Autodesk Inventor part; units mm, degrees
ref_plane "BODY_N_XY" through (79, 0, 0) normal (0, 0, -1) x (1, 0, 0)
ref_plane "BODY_N_YZ" through (79, 0, 0) normal (1, 0, 0) x (0, -1, 0)
ref_plane "BODY_N_ZX" through (79, 0, 0) normal (0, -1, 0) x (0, 0, -1)
sketch "Sketch_8" plane through (0, 0, 0) normal (0, 0, 1) x (1, 0, 0)
  line L0 (0, 0) -> (-8, 0)
  line L1 (-8, 0) -> (-8, 3.3865)
  line L2 (-8, 3.3865) -> (-7.3865, 4)
  line L3 (-7.3865, 4) -> (0, 4)
  line L4 (0, 4) -> (0, 0)
  line L5 (0, 0) -> (-8, 0)
revolve "Revolution1" add sketch "Sketch_8" angle 360 about axis through (0, 0, 0) along (1, 0, 0)
thread "Thread1"
sketch "Sketch_9" plane through (0, 0, 0) normal (1, 0, 0) x (0, 0, -1)
  line L0 (-6, 3.6056) -> (-6, -3.6056)
  arc A0 (-6, -3.6056) -> (-3.6056, -6) centre (0, 0) ccw
  line L1 (-3.6056, -6) -> (3.6056, -6)
  arc A1 (3.6056, -6) -> (6, -3.6056) centre (0, 0) ccw
  line L2 (6, -3.6056) -> (6, 3.6056)
  arc A2 (6, 3.6056) -> (3.6056, 6) centre (0, 0) ccw
  line L3 (3.6056, 6) -> (-3.6056, 6)
  arc A3 (-3.6056, 6) -> (-6, 3.6056) centre (0, 0) ccw
extrude "Extrusion1" add sketch "Sketch_9" along normal blind 12.5
sketch "Sketch_6" plane through (12.5, 0, 0) normal (1, 0, 0) x (0, 0, -1)
  circle A0 centre (0, 0) radius 5.5
extrude "Extrusion2" add sketch "Sketch_6" along normal blind 49
sketch "Sketch_10" plane through (61.5, 0, 0) normal (1, 0, 0) x (0, 0, -1)
  line L0 (-6, 3.6056) -> (-6, -3.6056)
  arc A0 (-6, -3.6056) -> (-3.6056, -6) centre (0, 0) ccw
  line L1 (-3.6056, -6) -> (3.6056, -6)
  arc A1 (3.6056, -6) -> (6, -3.6056) centre (0, 0) ccw
  line L2 (6, -3.6056) -> (6, 3.6056)
  arc A2 (6, 3.6056) -> (3.6056, 6) centre (0, 0) ccw
  line L3 (3.6056, 6) -> (-3.6056, 6)
  arc A3 (-3.6056, 6) -> (-6, 3.6056) centre (0, 0) ccw
extrude "Extrusion3" add sketch "Sketch_10" along normal blind 22.5
sketch "Sketch7" plane through (0, 0, 0) normal (0, 0, 1) x (1, 0, 0)
  line L0 (8, 6) -> (8, 1)
  line L1 (8, -0.1934) -> (5.933, 1)
  line L2 (5.933, 1) -> (5.933, 5.567)
  line L3 (5.933, 5.567) -> (5.5, 6)
  line L4 (5.5, 6) -> (8, 6)
  line L5 (8, 6) -> (8, -0.1934)
revolve "Revolution2" cut sketch "Sketch7" angle 360 about axis through (8, 6, 0) along (0, 1, 0)
thread "Thread2"
sketch "Sketch_7" plane through (0, 0, 0) normal (0, 0, 1) x (1, 0, 0)
  line L0 (66, 6) -> (66, 1)
  line L1 (66, -0.1934) -> (63.933, 1)
  line L2 (63.933, 1) -> (63.933, 5.567)
  line L3 (63.933, 5.567) -> (63.5, 6)
  line L4 (63.5, 6) -> (66, 6)
  line L5 (66, 6) -> (66, -0.1934)
revolve "Revolution3" cut sketch "Sketch_7" angle 360 about axis through (66, 6, 0) along (0, 1, 0)
thread "Thread3"
sketch "Sketch_16" plane through (0, 0, 0) normal (0, 0, 1) x (1, 0, 0)
  line L0 (42.5, 0) -> (-8, 0)
  line L1 (-8, 0) -> (-8, 2)
  line L2 (-8, 2) -> (12.5, 2)
  line L3 (12.5, 2) -> (12.5, 5)
  line L4 (12.5, 5) -> (42.5, 5)
  line L5 (42.5, 5) -> (42.5, 0)
  line L6 (42.5, 0) -> (-8, 0)
revolve "Revolution4" cut sketch "Sketch_16" angle 360 about axis through (42.5, 0, 0) along (1, 0, 0)
sketch "Sketch_3" plane through (0, 0, 0) normal (0, 1, 0) x (-1, 0, 0)
  line L0 (-71, 1.6) -> (-84, 1.6)
  line L1 (-84, 1.6) -> (-84, -1.6)
  line L2 (-84, -1.6) -> (-71, -1.6)
  line L3 (-71, -1.6) -> (-71, 1.6)
extrude "Extrusion4" cut sketch "Sketch_3" along normal mid plane 12
sketch "Sketch_13" plane through (0, 0, 0) normal (0, 0, 1) x (1, 0, 0)
  circle A0 centre (79, 0) radius 1.65
extrude "Extrusion5" cut sketch "Sketch_13" along normal mid plane 12
ref_plane "BODY_N_XY" through (79, 0, 0) normal (0, 0, -1) x (1, 0, 0)
ref_plane "BODY_N_YZ" through (79, 0, 0) normal (1, 0, 0) x (0, -1, 0)
ref_plane "BODY_N_ZX" through (79, 0, 0) normal (0, -1, 0) x (0, 0, -1)
ref_plane "BODY_PIN_XY" through (79, 0, 0) normal (-1, 0, 0) x (0, 0, -1)
ref_plane "BODY_PIN_YZ" through (79, 0, 0) normal (0, 0, -1) x (0, -1, 0)
ref_plane "BODY_PIN_ZX" through (79, 0, 0) normal (0, -1, 0) x (-1, 0, 0)
ref_plane "NUT2_XY" through (71, 0, 0) normal (1, 0, 0) x (0, 0, -1)
ref_plane "NUT2_YZ" through (71, 0, 0) normal (0, 0, -1) x (0, 1, 0)
ref_plane "NUT2_ZX" through (71, 0, 0) normal (0, 1, 0) x (1, 0, 0)
ref_plane "SW1_XY" through (17, 0, 0) normal (1, 0, 0) x (0, 0, -1)
ref_plane "SW1_YZ" through (17, 0, 0) normal (0, 0, -1) x (0, 1, 0)
ref_plane "SW1_ZX" through (17, 0, 0) normal (0, 1, 0) x (1, 0, 0)
ref_plane "SW2_XY" through (57, 0, 0) normal (-1, 0, 0) x (0, 0, -1)
ref_plane "SW2_YZ" through (57, 0, 0) normal (0, 0, -1) x (0, -1, 0)
ref_plane "SW2_ZX" through (57, 0, 0) normal (0, -1, 0) x (-1, 0, 0)
ref_plane "SW_R1_XY" through (17, -11, 0) normal (1, 0, 0) x (0, 0, -1)
ref_plane "SW_R1_YZ" through (17, -11, 0) normal (0, 0, -1) x (0, 1, 0)
ref_plane "SW_R1_ZX" through (17, -11, 0) normal (0, 1, 0) x (1, 0, 0)
ref_plane "SW_R2_XY" through (57, -11, 0) normal (-1, 0, 0) x (0, 0, -1)
ref_plane "SW_R2_YZ" through (57, -11, 0) normal (0, 0, -1) x (0, -1, 0)
ref_plane "SW_R2_ZX" through (57, -11, 0) normal (0, -1, 0) x (-1, 0, 0)
ref_plane "body_XY" through (0, 0, 0) normal (-1, 0, 0) x (0, 0, -1)
ref_plane "body_YZ" through (0, 0, 0) normal (0, 0, -1) x (0, -1, 0)
ref_plane "body_ZX" through (0, 0, 0) normal (0, -1, 0) x (-1, 0, 0)
properties part number "CJ2D10-25Z(1_0)_BODY"
Input: part model. Units: mm. Frame: model coordinates. A direction names the side the tool comes from. Coordinates: 2 decimals unless noted, no trailing zeros. Loops run counter-clockwise (first coordinate to the right, second up) from the corner with the lowest first, then second, coordinate; pieces in that order, holes last.
Q1. Contact query for flat-ended pins moving along their axis: pin 1 (3.5 mm diameter, centred on x = 66, z = 0, fed in from +Y); pin 2 (4 mm diameter, centred on x = 18, z = -1, fed in from -Y); pin 3 (3 mm diameter, centred on x = 79, y = 0, fed in from +Z); pin 4 (6 mm diameter, centred on x = 46, z = -2, fed in from +Y). Output: stop coordinate, or through.
Q2. Cut plane B-B (x = 58). Output: boundary loops of the cut face in (y, z).
Q3. Material intervals for line 1 (X direction, y = 0, z = 3.15); line 2 (Z direction, x = 8, y = 2.4); line 3 (X direction, y = 0, z = 3.95), sorted ascending.
Q4. Draft query along Z for faces 1 (the face through (77.35, -0.07, 3.77)), 2 (the face through (72.6, 5, -4.9)), 3 (the face through (27.71, -1.08, -4.88)), 4 (the face through (-3.642, -0.867, -3.905)). Return one class per face: +Z half, -Z half, draft (parallel to the pull), parting line (faces both ways), or undercut.
Q5. Set-up query: faces 5 (the face through (84, 0, 4)), 6 (the face through (61.5, -5, 3)), 7 (the face through (0, 4.1, 1.4)). Return all of +Z, -Z, +X, -X, +Y, -Y with unobstructed straight access to the full face (end or side cutting, diameter ignored); none if empty.
Q6. Cut plane A-A (x = 3). Output: boundary loops of the cut face in (y, z).
Q7. Cut plane C-C (x = 15). Output: boundary loops of the cut face in (y, z).
Working result:
1. pin 1: stops at y = 0.82
1. pin 2: stops at y = -5.5
1. pin 3: passes through
1. pin 4: stops at y = 5.5
2. outline: circle Ø11 at (0, 0)
3. line 1: x = -8 to 12.5, 42.5 to 77.35, 80.65 to 84
3. line 2: z = -6 to -2.07, 2.07 to 6
3. line 3: x = -7.44 to 12.5, 42.5 to 77.35, 80.65 to 84
4. face 1: draft
4. face 2: -Z half
4. face 3: undercut
4. face 4: parting line
5. face 5: +Z, -Z, +X, +Y, -Y
5. face 6: none
5. face 7: -X
6. outline: (-6, -3.61) arc R7 ccw to (-3.61, -6) - (3.61, -6) arc R7 ccw to (6, -3.61) - (6, 3.61) arc R7 ccw to (3.61, 6) - (-3.61, 6) arc R7 ccw to (-6, 3.61) - close; hole circle Ø4 at (0, 0)
7. outline: circle Ø11 at (0, 0); hole circle Ø10 at (0, 0)
